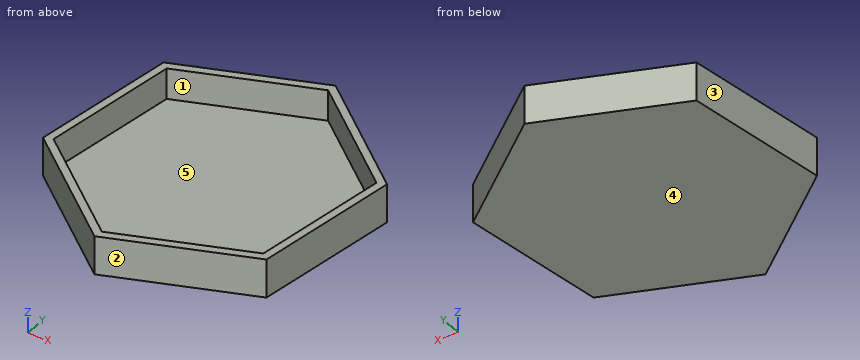
from build123d import *

# Parameters (mm, degrees)
F1_DEPTH = 25.4
F2_T     = -5.08


with BuildPart() as f1:
    # F0 (on Top) → F1 (new body)
    with BuildSketch(Plane.XY):
        Polygon((84.735168, -58.349015), (97.371386, 36.462443), (21.580365, 94.811458), (-66.846875, 58.349015), (-79.483094, -36.462443), (-3.692072, -94.811458), align=None)
    extrude(amount=F1_DEPTH)

    # F2
    f2_openings = [f1.faces().sort_by_distance(p)[0] for p in [
        (8.944146, 0, 25.4),
    ]]
    offset(amount=F2_T, openings=f2_openings)


solid = f1.part
Can you work these out from the model? Positions are in its coordinate system, mm. Face numbers are marked on the shaded views. A direction names the side the tool comes from. Give positions to 0.01 mm unless a question says otherwise; leave off trailing zeros. Loops run counter-clockwise (first coordinate to the right, second up) from the corner with the lowest first, then second, coordinate; pieces in that order, holes last. Notation, with made-up numbers: (15.25, -33) - (56.25, -33) arc R16 ccw to (56.25, -12) - close; hole circle Ø11 at (-4.5, -0.75). An arc over 180 degrees is marked (long way). Return JSON: item names as keys, results as strings.
1. For the marked faces 4 and 5, which set-ups out of +Z, -Z, +X, -X, +Y, -Y let a thin tool reach every point of the face, with its end or its side?
Output values:
{"face 4": "-Z, +X, -X, +Y, -Y", "face 5": "+Z"}
2. I'm going to push flat-ended pins straight in: pin 1 Ø8 at (y, z) = (-61, 15.5) entering from -X; pin 2 Ø5 at (y, z) = (57.5, 15) entering from -X; pin 3 Ø8 at (x, y) = (0.5, -59) entering from -Z; pin 4 Ø5 at (x, z) = (-36, 11.5) entering from +Y. Where does each tip first touch, or does it pass through?
Output values:
{"pin 1": "stops at x = -52.81", "pin 2": "stops at x = -67.29", "pin 3": "stops at z = 0", "pin 4": "stops at y = 72.1"}
3. I want a section at B-B on y = 50.5. Please give me the cut outline in (x, z).
Output values:
{"outline": "(-67.89, 0) - (79.14, 0) - (79.14, 25.4) - (70.81, 25.4) - (70.81, 5.08) - (-62.77, 5.08) - (-62.77, 25.4) - (-67.89, 25.4) - close"}
4. I want a section at C-C on x = 9. Please give me the cut outline in (y, z).
Output values:
{"outline": "(-89.58, 0) - (89.62, 0) - (89.62, 25.4) - (84.13, 25.4) - (84.13, 5.08) - (-84.08, 5.08) - (-84.08, 25.4) - (-89.58, 25.4) - close"}
5. I want a section at A-A on z = 8.5. Please give me the cut outline in (x, y), and give its area (3 significant figures).
Output values:
{"outline": "(-79.48, -36.46) - (-3.69, -94.81) - (84.74, -58.35) - (97.37, 36.46) - (21.58, 94.81) - (-66.85, 58.35) - close; hole (-74.06, -34.23) - (-2.92, -89) - (80.09, -54.77) - (91.95, 34.23) - (20.81, 89) - (-62.2, 54.77) - close", "area": "2,830 mm²"}
6. If I drill on line 1 (Z direction, x = 4, y = -84); line 2 (X direction, y = 86, z = 5.5); line 3 (X direction, y = -56.5, z = 17), over which ranges is the centre line in solid material (lowest first)?
Output values:
{"line 1": "z = 0 to 5.08", "line 2": "x = 0.21 to 13.54, 24.7 to 33.03", "line 3": "x = -53.46 to -45.13, 75.89 to 84.98"}
7. We'd pull the mould along X, two halves only. Please class the marked faces 1, 2 and 3: +X half, -X half, draft (parallel to the pull), parting line (faces both ways), or undercut.
Output values:
{"face 1": "undercut", "face 2": "+X half", "face 3": "-X half"}
